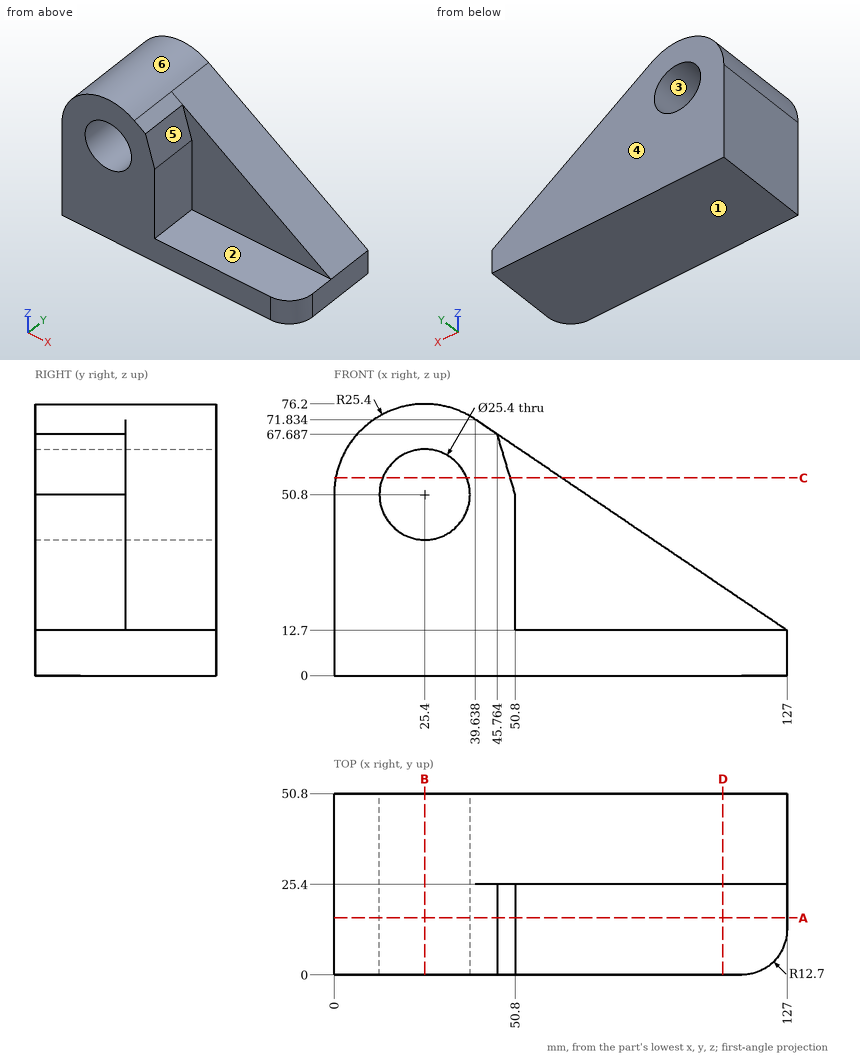
Can you work these out from the drawing? Everything is in mm from the part's minimum corner. A direction names the side the tool comes from. Round coordinates to 2 decimals unless told otherwise and drop trailing zeros. Order: outer loops, then holes, each group sorted by start corner. A loop starts at its lowest first (then second) coordinate and runs counter-clockwise, first axis right, second up. Notation, with made-up numbers: M 54,30 L 101,30 A7 cw 101,41 Z; hole C 18.5,68 d6. An arc over 180 degrees is marked long. One line per question, with ' | ' between items.
1) I want a section at A-A, the plane y = 16. Write out the boundary of the cut face in (x, z) (1 decimal).
Working result:
outline: M 0,0 L 127,0 L 127,12.7 L 50.8,12.7 L 50.8,50.8 L 45.8,67.7 L 39.6,71.8 A25.4 ccw 0,50.8 Z; hole C 25.4,50.8 d25.4
2) If we mould it in two halves opening along Z, with no side actions, what happens to the marked faces 1, 2, 3 and 4? For each: +Z half, -Z half, draft (parallel to the pull), parting line (faces both ways), or undercut.
Working result:
face 1: -Z half | face 2: +Z half | face 3: undercut | face 4: draft
3) I want a section at D-D, the plane x = 109. Write out the boundary of the cut face in (y, z).
Working result:
outline: M 0,0 L 50.8,0 L 50.8,24.88 L 25.4,24.88 L 25.4,12.7 L 0,12.7 Z
4) I need wall thicknesses on line 1 along Z through (x, y) = (25.4, 36); line 2 along Z through (x, y) = (101, 7.5); line 3 along X through (y, z) = (16, 50) (1 decimal). Which ranges of each line are inside material? Lowest first, please.
Working result:
line 1: 0 to 38.1, 63.5 to 76.2 | line 2: 0 to 12.7 | line 3: 0 to 12.7, 38.1 to 50.8
5) For pin 1 Ø3 at (x, y) = (77.5, 29.5) entering from +Z; pin 2 Ø20.5 at (x, y) = (77.5, 10) entering from +Z; pin 3 Ø1.5 at (x, z) = (59.5, 36) entering from -Y; pin 4 Ø10 at (x, y) = (25, 9.5) entering from +Z, each with a flat end and sliding along its axis, tell me the tip position at first contact or that it passes through.
Working result:
pin 1: z = 47.22 | pin 2: z = 12.7 | pin 3: y = 25.4 | pin 4: z = 76.2
6) I want a section at C-C, the plane z = 55.5. Write out the boundary of the cut face in (x, y), then the cut area to 3 significant figures.
Working result:
outline: M 0.44,0 L 13.6,0 L 13.6,50.8 L 0.44,50.8 Z; M 37.2,0 L 49.4,0 L 49.4,25.4 L 63.77,25.4 L 63.77,50.8 L 37.2,50.8 Z | area: 1,650 mm²
7) I want a section at B-B, the plane x = 25.4. Write out the boundary of the cut face in (y, z).
Working result:
outline: M 0,0 L 50.8,0 L 50.8,38.1 L 0,38.1 Z; M 0,63.5 L 50.8,63.5 L 50.8,76.2 L 0,76.2 Z
8) For the marked faces 5 and 6, which set-ups out of +Z, -Z, +X, -X, +Y, -Y let a thin tool reach every point of the face, with its end or its side?
Working result:
face 5: +Z, +X, -Y | face 6: +Z, +Y, -Y
